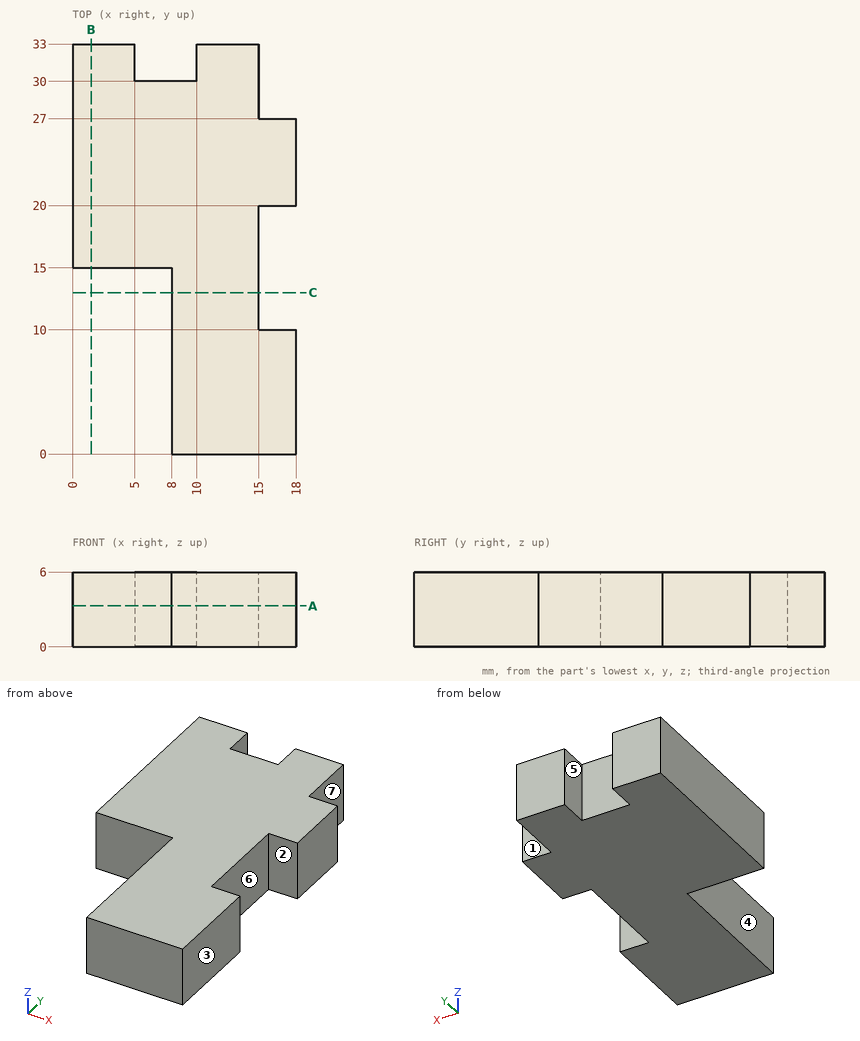
Input: dimensioned drawing with shaded views. Units: mm. Origin: part minimum x, y, z. A direction names the side the tool comes from. Round coordinates to 2 decimals unless told otherwise and drop trailing zeros. Order: outer loops, then holes, each group sorted by start corner. A loop starts at its lowest first (then second) coordinate and runs counter-clockwise, first axis right, second up.
1. Cut plane C-C, the plane y = 13. Output: boundary loops of the cut face in (x, z), then the cut area to 3 significant figures.
The answers:
outline: (8, 0) - (15, 0) - (15, 6) - (8, 6) - close
area: 42.0 mm2
2. Set-up query: the marked faces 4, 5, 6 and 7. Return all of +Z, -Z, +X, -X, +Y, -Y with unobstructed straight access to the full face (end or side cutting, diameter ignored); none if empty.
The answers:
face 4: +Z, -Z, -X, -Y
face 5: +Z, -Z, +Y
face 6: +Z, -Z, +X
face 7: +Z, -Z, +X, +Y
3. Mould query, pull axis Y, two halves, no side actions, for the marked faces 1, 2 and 3. Classes: released by +Y, released by -Y, zero draft, split by the parting line, or undercut.
The answers:
face 1: released by +Y
face 2: undercut
face 3: zero draft
4. Material intervals for line 1 (X direction, y = 31.5, z = 5.15); line 2 (X direction, y = 14.5, z = 4.45); line 3 (Y direction, x = 6.75, z = 5), sorted ascending.
The answers:
line 1: x = 0 to 5, 10 to 15
line 2: x = 8 to 15
line 3: y = 15 to 30
5. Cut plane A-A, the plane z = 3.3. Output: boundary loops of the cut face in (x, y), then the cut area to 3 significant figures.
The answers:
outline: (0, 15) - (8, 15) - (8, 0) - (18, 0) - (18, 10) - (15, 10) - (15, 20) - (18, 20) - (18, 27) - (15, 27) - (15, 33) - (10, 33) - (10, 30) - (5, 30) - (5, 33) - (0, 33) - close
area: 411 mm2
6. Cut plane B-B, the plane x = 1.5. Output: boundary loops of the cut face in (y, z), then the cut area to 3 significant figures.
The answers:
outline: (15, 0) - (33, 0) - (33, 6) - (15, 6) - close
area: 108 mm2
7. Pin query (flat end, axial travel): P1, Ø1.5, axis at y = 31.5, z = 4, coming from the +X side; P2, Ø2, axis at x = 2.5, z = 5.5, coming from the -Y side; P3, Ø3, axis at y = 8.5, z = 5.5, coming from the -X side. Return the tip coordinate at first contact, or that it passes through.
The answers:
P1: stops at x = 15
P2: stops at y = 15
P3: stops at x = 8
